For this review, take the finished solid that the model builds, in its own axes (mm). A direction names the side the tool comes from. Round coordinates to 2 decimals unless told otherwise and drop trailing zeros. Order: outer loops, then holes, each group sorted by start corner. A loop starts at its lowest first (then second) coordinate and runs counter-clockwise, first axis right, second up. Notation, with made-up numbers: (13, -11) - (60, -11) arc R25 ccw to (60, 5) - close; hole circle Ø11 at (37, 1). An arc over 180 degrees is marked (long way). Write each question's results on one line, items separated by ' | '. Start each with the question number.
(1) Take a section at B-B, the plane y = 2.55. Give the boundary of the cut face in (x, z) (3 decimals).
(2) Insertion check: pin 1 Ø3 at (x, z) = (-15, 1.5) entering from +Y. The pin has a flat end and moves straight along its axis. Give the tip position at first contact, or say it passes through.
(3) Take a section at C-C, the plane z = -0.5. Give the number of separate pieces and of enclosed holes in the cut face, plus the area to 4 significant figures.
(4) Take a section at A-A, the plane x = -18. Give the boundary of the cut face in (y, z) (3 decimals), plus the area to 4 significant figures.
(5) For L1, parallel to X at y = 2.05, z = -1 (3 decimals); L2, parallel to Z at x = -30, y = 2.1 (3 decimals); L3, parallel to X at y = 1.7, z = -4.5 (3 decimals), list the stretches that pass through material, from the lowest coordinate up. Write a range as from..to.
(6) For faces 1 (the flat face through (30.1, 1.5, -5.075)), 2 (the flat face through (35.6, 1, 0)), 3 (the flat face through (8, 0, 0)), list the 3-axis set-ups (+Z, -Z, +X, -X, +Y, -Y) from which the entire face can be reached by the end or side of a thin tool; tool diameter is ignored.
(7) Draft analysis for pull direction Z (two halves, no side actions). For faces 4 (the flat face through (8, 3, 0)), 5 (the flat face through (-14.8, 1.5, 5.075)), state which applies: pulls with the +Z half, pulls with the -Z half, needs draft (parallel to the pull), parting line crosses it, or undercut.
```python
from build123d import *

# Parameters (mm, degrees)
SKETCH1_W           = 76.1
SKETCH1_H           = 15
SKETCH1_W_2         = 10.75
SKETCH1_H_2         = 10.15
SKETCH1_W_3         = 10.7
SKETCH1_W_4         = 10.65
SKETCH1_W_5         = 10.6
SKETCH1_W_6         = 10.55
BOSS_EXTRUDE1_DEPTH = 3
SKETCH1_3_W         = 4
SKETCH1_3_H         = 10.15
BOSS_EXTRUDE2_DEPTH = 1
FILLET1_R           = 5
FILLET2_R           = 1


with BuildPart() as part:
    # Sketch1 → Boss-Extrude1 (new body)
    with BuildSketch(Plane(origin=(0, 0, 0), x_dir=(1, 0, 0), z_dir=(0, 1, 0))):
        Rectangle(SKETCH1_W, SKETCH1_H)
        with Locations((30.225, 0)):
            Rectangle(SKETCH1_W_2, SKETCH1_H_2, mode=Mode.SUBTRACT)
        with Locations((15.225, 0)):
            Rectangle(SKETCH1_W_3, SKETCH1_H_2, mode=Mode.SUBTRACT)
        with Locations((0.225, 0)):
            Rectangle(SKETCH1_W_4, SKETCH1_H_2, mode=Mode.SUBTRACT)
        with Locations((-14.775, 0)):
            Rectangle(SKETCH1_W_5, SKETCH1_H_2, mode=Mode.SUBTRACT)
        with Locations((-29.775, 0)):
            Rectangle(SKETCH1_W_6, SKETCH1_H_2, mode=Mode.SUBTRACT)
    extrude(amount=BOSS_EXTRUDE1_DEPTH)

    # Sketch1_3 → Boss-Extrude2 (add)
    with BuildSketch(Plane(origin=(0, 0, 0), x_dir=(1, 0, 0), z_dir=(0, 1, 0))):
        with Locations((-29.775, 0)):
            Rectangle(SKETCH1_3_W, SKETCH1_3_H)
        with Locations((-14.775, 0)):
            Rectangle(SKETCH1_3_W, SKETCH1_3_H)
        with Locations((0.225, 0)):
            Rectangle(SKETCH1_3_W, SKETCH1_3_H)
        with Locations((15.225, 0)):
            Rectangle(SKETCH1_3_W, SKETCH1_3_H)
        with Locations((30.225, 0)):
            Rectangle(SKETCH1_3_W, SKETCH1_3_H)
    extrude(amount=BOSS_EXTRUDE2_DEPTH)

    # Fillet1
    fillet1_edges = [part.edges().sort_by_distance(p)[0] for p in [
        (-38.05, 1.5, -7.5),
    ]]
    fillet(fillet1_edges, radius=FILLET1_R)

    # Fillet2
    fillet2_edges = [part.edges().sort_by_distance(p)[0] for p in [
        (-38.05, 1.5, 7.5),
        (38.05, 1.5, -7.5),
        (38.05, 1.5, 7.5),
    ]]
    fillet(fillet2_edges, radius=FILLET2_R)


solid = part.part
```
Results below:
1) outline: (-38.05, -2.5) arc R5 ccw to (-33.05, -7.5) - (37.05, -7.5) arc R1 ccw to (38.05, -6.5) - (38.05, 6.5) arc R1 ccw to (37.05, 7.5) - (-37.05, 7.5) arc R1 ccw to (-38.05, 6.5) - close; hole (-35.05, -5.075) - (-24.5, -5.075) - (-24.5, 5.075) - (-35.05, 5.075) - close; hole (-20.075, -5.075) - (-9.475, -5.075) - (-9.475, 5.075) - (-20.075, 5.075) - close; hole (-5.1, -5.075) - (5.55, -5.075) - (5.55, 5.075) - (-5.1, 5.075) - close; hole (9.875, -5.075) - (20.575, -5.075) - (20.575, 5.075) - (9.875, 5.075) - close; hole (24.85, -5.075) - (35.6, -5.075) - (35.6, 5.075) - (24.85, 5.075) - close
2) pin 1: stops at y = 1
3) separate pieces: 11 | enclosed holes: 0 | area: 88.55 mm^2
4) outline: (0, -7.5) - (3, -7.5) - (3, -5.075) - (0, -5.075) - close; (0, 5.075) - (3, 5.075) - (3, 7.5) - (0, 7.5) - close | area: 14.55 mm^2
5) L1: x = -38.05..-35.05, -24.5..-20.075, -9.475..-5.1, 5.55..9.875, 20.575..24.85, 35.6..38.05 | L2: z = -7.5..-5.075, 5.075..7.5 | L3: x = -37.633..-35.05, -24.5..-20.075, -9.475..-5.1, 5.55..9.875, 20.575..24.85, 35.6..38.05
6) face 1: +Y | face 2: +Y, -Y | face 3: +Z, -Z, +X, -X, -Y
7) face 4: needs draft | face 5: undercut
